```python
from build123d import *

# Parameters (mm, degrees)
BOSS_EXTRUDE1_DEPTH         = 3
SKETCH1_4_W                 = 3
SKETCH1_4_H                 = 20
BOSS_EXTRUDE3_DEPTH         = 55
M8_CLEARANCE_HOLE1_D        = 9
TAP_DRILL_FOR_M3X0_5_TAP1_D = 2.5
FILLET1_R                   = 5


with BuildPart() as part:
    # Sketch1 → Boss-Extrude1 (new body)
    with BuildSketch(Plane(origin=(0, 0, 0), x_dir=(1, 0, 0), z_dir=(0, 1, 0))):
        with BuildLine():
            Line((-12.5, -12.5), (0, -12.5))
            ThreePointArc((0, -12.5), (11.180339887, 5.590169944), (-10, 7.5))
            Line((-10, 7.5), (-12.5, 7.5))
            Line((-12.5, 7.5), (-12.5, -12.5))
        make_face()
    extrude(amount=BOSS_EXTRUDE1_DEPTH)

    # Sketch1<4> → Boss-Extrude3 (add)
    with BuildSketch(Plane(origin=(0, 0, 0), x_dir=(1, 0, 0), z_dir=(0, 1, 0))):
        with Locations((-11, -2.5)):
            Rectangle(SKETCH1_4_W, SKETCH1_4_H)
    extrude(amount=BOSS_EXTRUDE3_DEPTH)

    # M8 Clearance Hole1 (through all)
    with Locations(Plane(origin=(0, 0, 0), x_dir=(-1, 0, 0), z_dir=(0, -1, 0))):
        with Locations((0, 0)):
            Hole(M8_CLEARANCE_HOLE1_D / 2)

    # Tap Drill for M3x0.5 Tap1 (through all)
    with Locations(Plane.ZY.offset(12.5)):
        with Locations((2.5, 27)):
            Hole(TAP_DRILL_FOR_M3X0_5_TAP1_D / 2)

    # Fillet1
    # the kernel refuses this fillet: 5 mm, written as the material it takes off along each edge
    with BuildSketch(Plane(origin=(-12.5, -12.5, 12.5), x_dir=(0, 0, -1), z_dir=(0, 1, 0))) as fillet1_piece_1:
        with BuildLine():
            CenterArc((FILLET1_R, -FILLET1_R), FILLET1_R, 90, 90)
            Line((0, -FILLET1_R), (0, 0))
            Line((0, 0), (FILLET1_R, 0))
        make_face()
    extrude(amount=80, mode=Mode.SUBTRACT)
    with BuildSketch(Plane(origin=(-12.5, -11.456439237, -7.5), x_dir=(1, 0, 0), z_dir=(0, 1, 0))) as fillet1_piece_2_section:
        with BuildLine():
            CenterArc((5, -4.582575695), FILLET1_R, 113.578178478, 66.421821522)
            Line((0, -4.582575695), (0, 0))
            Line((0, 0), (3, 0))
        make_face()
    fillet1_piece_2 = extrude(amount=77.912878475, mode=Mode.PRIVATE)
    fillet1_piece_2 = fillet1_piece_2 - Plane(origin=(0, -11.456439237, 0), x_dir=(0, 0, 1), z_dir=(0, -1, 0)) * Cylinder(12.5, 175, mode=Mode.PRIVATE)
    add(fillet1_piece_2, mode=Mode.SUBTRACT)
    with BuildSketch(Plane(origin=(-12.5, -11.456439237, -7.5), x_dir=(1, 0, 0), z_dir=(0, 1, 0))) as fillet1_piece_3_section:
        with BuildLine():
            CenterArc((5, -4.582575695), FILLET1_R, 113.578178478, 66.421821522)
            Line((0, -4.582575695), (0, 0))
            Line((0, 0), (3, 0))
        make_face()
    fillet1_piece_3 = extrude(amount=77.912878475, mode=Mode.PRIVATE)
    fillet1_piece_3 = split(fillet1_piece_3, bisect_by=Plane(origin=(-12.5, 3, -7.5), z_dir=(0, 1, 0)), keep=Keep.TOP, mode=Mode.PRIVATE)
    add(fillet1_piece_3, mode=Mode.SUBTRACT)


solid = part.part
```
CAD build for the part. Positions are in the model's coordinates, mm. Round coordinates to 2 decimals unless told otherwise and drop trailing zeros. Order: outer loops, then holes, each group sorted by start corner. A loop starts at its lowest first (then second) coordinate and runs counter-clockwise, first axis right, second up.
Item 1: Mould opens along Z. For faces 1 (the face through (-11.66, 27.11, -5.69)), 2 (the face through (-0.59, 1.52, -4.46)), 3 (the face through (-9.5, 29, 2)) say: pulls with the +Z half, pulls with the -Z half, needs draft (parallel to the pull), parting line crosses it, or undercut.
Item 2: Saw through at B-B on z = 0. Write the cut outline in (x, y).
Item 3: Saw through at C-C on x = 2.5. Write the cut outline in (y, z).
Item 4: Probe line 1 along Y through (x, z) = (-11.75, 2.5); line 2 along Z through (x, y) = (0, 0.95); line 3 along X through (y, z) = (7.5, -3). List the from-to ranges inside material, lowest first.
Item 5: Saw through at D-D on z = 2.5. Write the cut outline in (x, y), then the cut area to 3 significant figures.
Item 6: Saw through at A-A on y = 27. Write the cut outline in (x, z).
Item 7: Pin check, flat tips, straight feed: pin 1 (11.5 mm diameter, centred on x = 0.5, z = 3, fed in from +Y); pin 2 (1.5 mm diameter, centred on y = 16, z = 2, fed in from +X); pin 3 (8 mm diameter, centred on x = 0, z = 0, fed in from -Y). Stop position of each tip, or through.
Reported:
1. face 1: pulls with the -Z half
1. face 2: undercut
1. face 3: needs draft
2. outline: (-12.5, 0) - (-4.5, 0) - (-4.5, 3) - (-9.5, 3) - (-9.5, 55) - (-12.5, 55) - close; (4.5, 0) - (12.5, 0) - (12.5, 3) - (4.5, 3) - close
3. outline: (0, -12.25) - (3, -12.25) - (3, -3.74) - (0, -3.74) - close; (0, 3.74) - (3, 3.74) - (3, 12.25) - (0, 12.25) - close
4. line 1: y = 0 to 25.75, 28.25 to 55
4. line 2: z = -12.5 to -4.5, 4.5 to 12.5
4. line 3: x = -12.5 to -9.5
5. outline: (-12.5, 0) - (-3.74, 0) - (-3.74, 3) - (-9.5, 3) - (-9.5, 25.75) - (-12.5, 25.75) - close; (-12.5, 28.25) - (-9.5, 28.25) - (-9.5, 55) - (-12.5, 55) - close; (3.74, 0) - (12.25, 0) - (12.25, 3) - (3.74, 3) - close
5. area: 200 mm2
6. outline: (-12.5, -2.92) arc R5 ccw to (-9.5, -7.5) - (-9.5, 1.25) - (-12.5, 1.25) - close; (-12.5, 3.75) - (-9.5, 3.75) - (-9.5, 12.08) arc R5 ccw to (-12.5, 7.5) - close
7. pin 1: stops at y = 3
7. pin 2: stops at x = -9.5
7. pin 3: passes through
